Autodesk Inventor part; units mm, degrees
ref_plane "YZ Plane" through (0, 0, 0) normal (1, 0, 0) x (0, 1, 0)
ref_plane "XZ Plane" through (0, 0, 0) normal (0, 1, 0) x (-1, 0, 0)
ref_plane "XY Plane" through (0, 0, 0) normal (0, 0, 1) x (1, 0, 0)
sketch "Sketch1" plane through (0, 0, 0) normal (1, 0, 0) x (0, 1, 0)
  line L0 (0, 0) -> (-38.1, 7.674)
  line L1 (-38.1, 7.674) -> (-38.1, 0)
  line L2 (-38.1, 0) -> (0, 0)
  dimension "d0" = 38.1
  dimension "d1" = 11.388
extrude "Extrusion1" add sketch "Sketch1" along normal blind 38.1
sketch "Sketch2" plane through (0, -38.1, 0) normal (0, 0, -1) x (-1, 0, 0)
  circle A0 centre (-19.05, 19.05) radius 19.05
  line L0 (0, 38.1) -> (-38.1, 38.1)
  line L1 (0, 0) -> (0, 38.1)
  line L2 (-38.1, 0) -> (-38.1, 38.1)
  circle A1 centre (-19.05, 19.05) radius 6.35
  point P0 (-38.1, 19.05)
  point P1 (-19.05, 38.1)
  point P2 (0, 19.05)
  dimension "d4" = 12.7
extrude "Extrusion2" cut sketch "Sketch2" against normal through all contours A0 L0 L1 | A0 L2 L0 | A1
fillet "Fillet1" radius 6.35 2 edges at (38.1, -38.1, 3.837) (0, -38.1, 3.837)
properties part number "TRI_SPACER_TOP_TREBUCHET" material "Wood (Birch)"
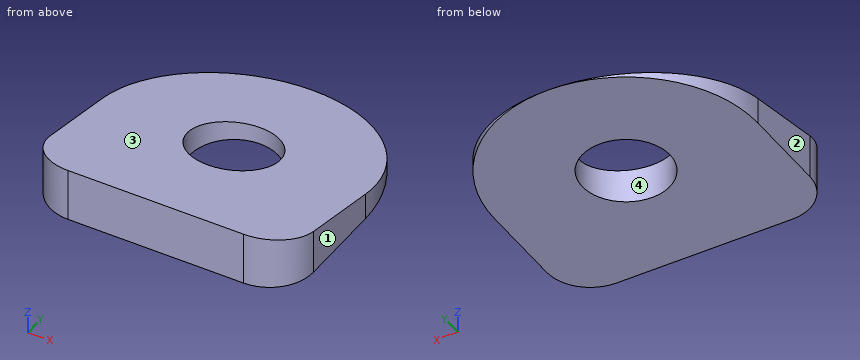
The listing builds one solid part. Answer for the finished solid, in the listing's coordinates (mm). Face numbers are marked on the shaded views. Round coordinates to 2 decimals unless told otherwise and drop trailing zeros. Loops run counter-clockwise (first coordinate to the right, second up) from the corner with the lowest first, then second, coordinate; pieces in that order, holes last. Notation, with made-up numbers: (-18, -9.5) -> (32, -9.5) arc R13 cw to (32, -4.5) -> close; hole circle Ø4 at (32, 82.25). An arc over 180 degrees is marked (long way). Use one line per item in the form item = value.
1. Flat-ended cylindrical pins translate along their axes: pin 1 Ø8 at (x, y) = (9, -32.5) entering from -Z; pin 2 Ø4 at (x, y) = (33.5, -24) entering from +Z; pin 3 Ø8 at (x, y) = (5, -29.5) entering from +Z; pin 4 Ø10 at (x, y) = (19.05, -19.05) entering from +Z (3 decimals). Find the tip coordinate at first contact, or state that the pin passes through.
Answer key:
pin_1 = 0
pin_2 = 5.24
pin_3 = 6.75
pin_4 = through
2. The part is cut by section B-B on z = 1. Determine the outline of the cut face in (x, y).
Answer key:
outline = (0, -31.75) arc R6.35 ccw to (6.35, -38.1) -> (31.75, -38.1) arc R6.35 ccw to (38.1, -31.75) -> (38.1, -19.05) arc R19.05 ccw to (31.88, -4.96) -> (6.22, -4.96) arc R19.05 ccw to (0, -19.05) -> close; hole circle Ø12.7 at (19.05, -19.05)
3. The part is cut by section C-C on y = -14.5. Determine the outline of the cut face in (x, z).
Answer key:
outline = (0.55, 0) -> (14.62, 0) -> (14.62, 2.92) -> (0.55, 2.92) -> close; (23.48, 0) -> (37.55, 0) -> (37.55, 2.92) -> (23.48, 2.92) -> close
4. For a pull along X with two mould halves and no side action, classify the marked faces 1, 2, 3 and 4 as released by +X, released by -X, zero draft, split by the parting line, or undercut.
Answer key:
face_1 = released by +X
face_2 = released by -X
face_3 = zero draft
face_4 = undercut
5. The part is cut by section D-D on z = 4.5. Determine the outline of the cut face in (x, y).
Answer key:
outline = (0, -31.75) arc R6.35 ccw to (6.35, -38.1) -> (31.75, -38.1) arc R6.35 ccw to (38.1, -31.75) -> (38.1, -22.34) -> (24.48, -22.34) arc R6.35 cw to (13.62, -22.34) -> (0, -22.34) -> close
6. The part is cut by section A-A on x = 14.5. Determine the outline of the cut face in (y, z), and give its area (3 significant figures).
Answer key:
outline = (-38.1, 0) -> (-23.48, 0) -> (-23.48, 4.73) -> (-38.1, 7.67) -> close; (-14.62, 0) -> (-0.55, 0) -> (-0.55, 0.11) -> (-14.62, 2.94) -> close
area = 112 mm²
7. Find the intervals of material crossed by probe 1 along X at (y, z) = (-19.05, 2.9); probe 2 along Y at (x, z) = (19.05, 3.75); probe 3 along X at (y, z) = (-16, 2.75), in increasing order. Write a range as [from, to].
Answer key:
probe_1 = [0, 12.7], [25.4, 38.1]
probe_2 = [-38.1, -25.4]
probe_3 = [0.25, 13.48], [24.62, 37.85]
